from build123d import *

# Parameters (mm, degrees)
SKETCH1_R           = 20
BOSS_EXTRUDE1_DEPTH = 165
SKETCH2_R           = 10
BOSS_EXTRUDE2_DEPTH = 40
SKETCH5_R           = 20
BOSS_EXTRUDE3_DEPTH = 150
SKETCH6_W           = 10
SKETCH6_H           = 34.641016151
BOSS_EXTRUDE5_DEPTH = 50
SKETCH7_R           = 5
CUT_EXTRUDE1_DEPTH  = 10


with BuildPart() as part:
    # Sketch1 → Boss-Extrude1 (new body)
    with BuildSketch(Plane(origin=(0, 0, 0), x_dir=(0, 0, -1), z_dir=(1, 0, 0))):
        Circle(SKETCH1_R)
    extrude(amount=BOSS_EXTRUDE1_DEPTH)

    # Sketch2 → Boss-Extrude2 (add)
    with BuildSketch(Plane(origin=(165, 0, 0), x_dir=(0, 0, -1), z_dir=(1, 0, 0))):
        Circle(SKETCH2_R)
    extrude(amount=BOSS_EXTRUDE2_DEPTH)

    # Sketch5 → Boss-Extrude3 (add)
    with BuildSketch(Plane(origin=(20, 20, 0), x_dir=(0.7071067811865464, -0.7071067811865488, 0), z_dir=(0.7071067811865488, 0.7071067811865464, 0))):
        with Locations(Location((28.284271247, 0, 0), (0, 0, 90))):
            Circle(SKETCH5_R)
    extrude(amount=BOSS_EXTRUDE3_DEPTH)

    # Sketch6 → Boss-Extrude5 (add)
    with BuildSketch(Plane(origin=(126.066017178, 126.066017178, 0), x_dir=(0, 0, -1), z_dir=(0.7071067811865487, 0.7071067811865465, 0))):
        with Locations((-5, -28.284271248)):
            Rectangle(SKETCH6_W, SKETCH6_H)
    extrude(amount=BOSS_EXTRUDE5_DEPTH)

    # Sketch7 → Cut-Extrude1 (cut)
    with BuildSketch(Plane.ZY):
        Circle(SKETCH7_R)
    extrude(amount=-CUT_EXTRUDE1_DEPTH, mode=Mode.SUBTRACT)


solid = part.part
For this review, take the finished solid that the model builds, in its own axes (mm). A direction names the side the tool comes from. Coordinates: 2 decimals unless noted, no trailing zeros. Loops run counter-clockwise (first coordinate to the right, second up) from the corner with the lowest first, then second, coordinate; pieces in that order, holes last. Notation, with made-up numbers: (-35.75, 52) - (15.25, 52) arc R21 ccw to (15.25, 76) - close; hole circle Ø5 at (-7, 46.25). An arc over 180 degrees is marked (long way). Use a Markdown table: item, result. Add a question column.
Item 1: Insertion check: pin 1 Ø12 at (x, z) = (151.5, 13) entering from +Y; pin 2 Ø3 at (y, z) = (-2, 0.5) entering from -X; pin 3 Ø2 at (y, z) = (92.5, -9) entering from -X; pin 4 Ø12 at (x, z) = (173, -4.5) entering from +Y. Each pin has a flat end and moves straight along its axis. Give the tip position at first contact, or say it passes through.
Item 2: For line 1 (Y direction, x = 8, z = 0); line 2 (Y direction, x = 85, z = -10); line 3 (X direction, y = 10, z = 8), list the stretches that pass through material, from the lowest coordinate up.
Item 3: We need section B-B (x = 25). Give the boundary of the cut face in (y, z).
Item 4: Tool access review of faces 5 (the face through (184.72, -9.76, 2.17)), 6 (the face through (205, 0, 0)), 7 (the face through (164, 123, 10)), 8 (the face through (175.744, 111.249, 5.07)): name each direction out of +Z, -Z, +X, -X, +Y, -Y from which nothing blocks a thin tool from reaching the whole face with its end or side.
Item 5: We need section A-A (z = -14). Give the boundary of the cut face in (x, y).
Item 6: Mouldability with a two-part tool opening along Z and no side actions: class faces 1 (the face through (4.93, -4.88, -1.08)), 2 (the face through (10, 0, 0)), 3 (the face through (164, 123, 0)), 4 (the face through (145.89, 106.24, 13.96)) as pulls with the +Z half, pulls with the -Z half, needs draft (parallel to the pull), parting line crosses it, or undercut.
Item 7: We need section C-C (z = 17.5). Give the boundary of the cut face in (x, y), and give its area (3 significant figures).
Results list:
| question | item | result |
|---|---|---|
| 1 | pin 1 | stops at y = 141.19 |
| 1 | pin 2 | stops at x = 10 |
| 1 | pin 3 | stops at x = 106.03 |
| 1 | pin 4 | stops at y = 153.67 |
| 2 | line 1 | y = -20 to -5, 5 to 20 |
| 2 | line 2 | y = -17.32 to 17.32, 20.51 to 69.49 |
| 2 | line 3 | x = 0 to 165 |
| 3 | outline | circle Ø40 at (0, 0) |
| 4 | face 5 | +X |
| 4 | face 6 | +Z, -Z, +X, +Y, -Y |
| 4 | face 7 | +Z, +X, +Y |
| 4 | face 8 | +Z, -Z, +X |
| 5 | outline | (0, -14.28) - (165, -14.28) - (165, 14.28) - (74.48, 14.28) - (156.17, 95.97) - (135.97, 116.17) - (34.08, 14.28) - (0, 14.28) - close |
| 6 | face 1 | undercut |
| 6 | face 2 | undercut |
| 6 | face 3 | pulls with the -Z half |
| 6 | face 4 | needs draft |
| 7 | outline | (0, -9.68) - (165, -9.68) - (165, 9.68) - (63.38, 9.68) - (152.91, 99.22) - (139.22, 112.91) - (35.99, 9.68) - (0, 9.68) - close |
| 7 | area | 5,830 mm^2 |
